Autodesk Inventor part; units mm, degrees
ref_plane "YZ Plane" through (0, 0, 0) normal (1, 0, 0) x (0, 1, 0)
ref_plane "XZ Plane" through (0, 0, 0) normal (0, 1, 0) x (-1, 0, 0)
ref_plane "XY Plane" through (0, 0, 0) normal (0, 0, 1) x (1, 0, 0)
sketch "Sketch1" plane through (0, 0, 0) normal (0, 0, 1) x (1, 0, 0)
  circle A0 centre (0, 0) radius 2
  dimension "d0" = 4
extrude "Extrusion1" add sketch "Sketch1" along normal mid plane 100
sketch "Sketch2" plane through (0, 0, 50) normal (0, 0, 1) x (1, 0, 0)
  circle A0 centre (0, 0) radius 8.069
extrude "Extrusion2" add sketch "Sketch2" against normal blind 5
sketch "Sketch3" plane through (0, 0, -50) normal (0, 0, -1) x (-1, 0, 0)
  circle A0 centre (0, 0) radius 8.069
extrude "Extrusion3" add sketch "Sketch3" against normal blind 5
properties part number "weights"
For this review, take the finished solid that the model builds, in its own axes (mm). A direction names the side the tool comes from. Round coordinates to 2 decimals unless told otherwise and drop trailing zeros. Loops run counter-clockwise (first coordinate to the right, second up) from the corner with the lowest first, then second, coordinate; pieces in that order, holes last. Notation, with made-up numbers: (-7.75, 65.5) - (23.25, 65.5) arc R30 ccw to (23.25, 87.5) - close; hole circle Ø10 at (-39.75, -39.5). An arc over 180 degrees is marked (long way). Answer as CSV lines item,"result".
(1) Consider section A-A on y = 6.5. Give the boundary of the cut face in (x, z).
Checked values:
outline,"(-4.78, -50) - (4.78, -50) - (4.78, -45) - (-4.78, -45) - close; (-4.78, 45) - (4.78, 45) - (4.78, 50) - (-4.78, 50) - close"
(2) Consider section B-B on y = 0. Give the boundary of the cut face in (x, z).
Checked values:
outline,"(-8.07, -50) - (8.07, -50) - (8.07, -45) - (2, -45) - (2, 45) - (8.07, 45) - (8.07, 50) - (-8.07, 50) - (-8.07, 45) - (-2, 45) - (-2, -45) - (-8.07, -45) - close"
(3) Mouldability with a two-part tool opening along Z and no side actions: class faces 1 (the face through (0, 0, 50)), 2 (the face through (-2, -2, -45)), 3 (the face through (-1.749, -7.877, 47.535)) as +Z half, -Z half, draft (parallel to the pull), parting line (faces both ways), or undercut.
Checked values:
face 1,"+Z half"
face 2,"undercut"
face 3,"draft"
(4) Consider section D-D on z = 30. Give the boundary of the cut face in (x, y), then the cut area to 3 significant figures.
Checked values:
outline,"circle Ø4 at (0, 0)"
area,"12.6 mm2"
(5) Insertion check: P1, Ø4, axis at y = -2.5, z = -37.5, coming from the +X side; P2, Ø1, axis at y = -2, z = 3.5, coming from the -X side; P3, Ø5, axis at y = -1, z = -35, coming from the -X side. Each pin has a flat end and moves straight along its axis. Give the tip position at first contact, or say it passes through.
Checked values:
P1,"stops at x = 1.94"
P2,"stops at x = -1.32"
P3,"stops at x = -2"
(6) Tool access review of faces 4 (the face through (0, 2, -1)), 5 (the face through (0, 0, -50)): name each direction out of +Z, -Z, +X, -X, +Y, -Y from which nothing blocks a thin tool from reaching the whole face with its end or side.
Checked values:
face 4,"none"
face 5,"-Z, +X, -X, +Y, -Y"
(7) Wall thickness on line 1 (Z direction, x = -4.25, y = -4.75); line 2 (X direction, y = 0.25, z = -9); line 3 (X direction, y = -1.75, z = 0.5): over which ranges is each line inside the solid? List them lowest first.
Checked values:
line 1,"z = -50 to -45, 45 to 50"
line 2,"x = -1.98 to 1.98"
line 3,"x = -0.97 to 0.97"
